```python
from build123d import *

# Parameters (mm, degrees)
EXTRUDE_1_DEPTH = 22
SKETCH_2_W      = 180
SKETCH_2_H      = 90
EXTRUDE_2_DEPTH = 1
SKETCH_3_W      = 10
SKETCH_3_H      = 5
EXTRUDE_3_DEPTH = 30
FILLET_1_R      = 10


with BuildPart() as part:
    # Эскиз1 → Бобышка-Вытянуть1 (new body)
    with BuildSketch(Plane(origin=(0, 0, 0), x_dir=(-1, 0, 0), z_dir=(0, 1, 0))):
        with BuildLine():
            Line((-90, 0), (90, 0))
            Line((90, 0), (90, 90))
            Line((90, 90), (81, 90))
            ThreePointArc((81, 90), (0, 9), (-81, 90))
            Line((-81, 90), (-90, 90))
            Line((-90, 90), (-90, 0))
        make_face()
    extrude(amount=EXTRUDE_1_DEPTH)

    # Эскиз2 → Бобышка-Вытянуть2 (add)
    with BuildSketch(Plane(origin=(0, 22, 0), x_dir=(1, 0, 0), z_dir=(0, 1, 0))):
        with Locations((0, -45)):
            Rectangle(SKETCH_2_W, SKETCH_2_H)
    extrude(amount=-EXTRUDE_2_DEPTH)

    # Эскиз3 → Бобышка-Вытянуть3 (add)
    with BuildSketch(Plane.XZ):
        with Locations((-85, 2.5)):
            Rectangle(SKETCH_3_W, SKETCH_3_H)
        with Locations((85, 2.5)):
            Rectangle(SKETCH_3_W, SKETCH_3_H)
    extrude(amount=EXTRUDE_3_DEPTH)

    # Скругление1
    fillet_1_edges = [part.edges().sort_by_distance(p)[0] for p in [
        (-80, 0, 2.5),
        (80, 0, 2.5),
    ]]
    fillet(fillet_1_edges, radius=FILLET_1_R)


solid = part.part
```
Could you check a few things on this model? Use its own coordinates, in mm. A direction names the side the tool comes from. Give positions to 0.01 mm unless a question says otherwise; leave off trailing zeros. Write each loop counter-clockwise with the first axis right and the second up, starting at its lowest first coordinate (ties: lowest second). Pieces come first, ordered by that corner, then holes. Notation, with made-up numbers: (-26, 7.5) -> (0, 7.5) arc R29 ccw to (0, 38.5) -> close; hole circle Ø8 at (53, 21.5). An arc over 180 degrees is marked (long way). Write each question's results on one line, items separated by ' | '.
1. I want a section at A-A, the plane y = -2. Write out the boundary of the cut face in (x, z).
Check sheet entries:
outline: (-90, 0) -> (-76, 0) -> (-76, 5) -> (-90, 5) -> close; (76, 0) -> (90, 0) -> (90, 5) -> (76, 5) -> close
2. Will these pins go through, and if not, where does the flat tip stop? pin 1 Ø1.5 at (x, z) = (25.5, 29.5) entering from -Y; pin 2 Ø22 at (x, y) = (-82.5, -19) entering from +Z.
Check sheet entries:
pin 1: stops at y = 21 | pin 2: stops at z = 5
3. On a 3-axis mill with a long thin cutter (end or side, diameter ignored), from which of +Z, -Z, +X, -X, +Y, -Y can I reach the whole of each face in a straight line? I mean faces 1 (the flat face through (90, 13, 46)), 2 (the flat face through (-85, -15, 5)), 3 (the flat face through (-80, -20, 2)), 4 (the cylindrical face through (-1.78, 10.35, 9.02)). Say none if no direction works.
Check sheet entries:
face 1: +Z, -Z, +X, +Y, -Y | face 2: +Z, +X, -X, -Y | face 3: +Z, -Z, -Y | face 4: +Z, -Y
4. I want a section at C-C, the plane y = 15. Write out the boundary of the cut face in (x, z).
Check sheet entries:
outline: (-90, 0) -> (90, 0) -> (90, 90) -> (81, 90) arc R81 cw to (-81, 90) -> (-90, 90) -> close
5. I want a section at B-B, the plane z = 34.5. Write out the boundary of the cut face in (x, y), then the cut area to 3 significant figures.
Check sheet entries:
outline: (-90, 0) -> (-59, 0) -> (-59, 21) -> (59, 21) -> (59, 0) -> (90, 0) -> (90, 22) -> (-90, 22) -> close | area: 1,480 mm²
6. I want a section at D-D, the plane x = 0. Write out the boundary of the cut face in (y, z), then the cut area to 3 significant figures.
Check sheet entries:
outline: (0, 0) -> (22, 0) -> (22, 90) -> (21, 90) -> (21, 9) -> (0, 9) -> close | area: 279 mm²
7. If we mould it in two halves opening along X, with no side actions, what happens to faces 5 (the flat face through (84, -15, 5)), 6 (the cylindrical face through (-77.15, -3.01, 2.54)), 7 (the flat face through (-90, 8, 44))? For each: released by +X, released by -X, zero draft, split by the parting line, or undercut.
Check sheet entries:
face 5: zero draft | face 6: undercut | face 7: released by -X
8. I need wall thicknesses on L1, parallel to X at y = 12, z = 74; L2, parallel to Y at x = -53, z = 35.5; L3, parallel to Y at x = -57, z = 7. Which ranges of each line are inside material? Lowest first, please.
Check sheet entries:
L1: x = -90 to -79.4, 79.4 to 90 | L2: y = 21 to 22 | L3: y = 0 to 22
